from build123d import *

# Parameters (mm, degrees)
F0_R     = 6.35
F1_DEPTH = 4.7498
F2_R     = 3.175
F3_DEPTH = 25.4
F5_DEPTH = 0.381
F7_DEPTH = 0.381


with BuildPart() as f1:
    # F0 (on Right) → F1 (new body)
    with BuildSketch(Plane.YZ):
        Circle(F0_R)
    extrude(amount=F1_DEPTH)

    # F2 (on face) → F3 (cut)
    with BuildSketch(Plane.YZ.offset(4.7498)):
        Circle(F2_R)
    extrude(amount=-F3_DEPTH, mode=Mode.SUBTRACT)

    # F4 (on face) → F5 (cut)
    with BuildSketch(Plane(origin=(0, 0, 0), x_dir=(0, -1, 0), z_dir=(-1, 0, 0))):
        with BuildLine():
            ThreePointArc((0, -5.969), (4.22072, -4.22072), (5.969, 0))
            ThreePointArc((5.969, 0), (4.22072, 4.22072), (0, 5.969))
            ThreePointArc((0, 5.969), (-5.969, 0), (0, -5.969))
        make_face()
        with BuildLine():
            ThreePointArc((0, 3.556), (2.514472, 2.514472), (3.556, 0))
            ThreePointArc((3.556, 0), (2.514472, -2.514472), (0, -3.556))
            ThreePointArc((0, -3.556), (-3.556, 0), (0, 3.556))
        make_face(mode=Mode.SUBTRACT)
    extrude(amount=-F5_DEPTH, mode=Mode.SUBTRACT)

    # F6 (on face) → F7 (cut)
    with BuildSketch(Plane.YZ.offset(4.7498)):
        with BuildLine():
            ThreePointArc((0, -5.969), (4.22072, -4.22072), (5.969, 0))
            ThreePointArc((5.969, 0), (4.22072, 4.22072), (0, 5.969))
            ThreePointArc((0, 5.969), (-5.969, 0), (0, -5.969))
        make_face()
        with BuildLine():
            ThreePointArc((0, 3.556), (2.514472, 2.514472), (3.556, 0))
            ThreePointArc((3.556, 0), (2.514472, -2.514472), (0, -3.556))
            ThreePointArc((0, -3.556), (-3.556, 0), (0, 3.556))
        make_face(mode=Mode.SUBTRACT)
    extrude(amount=-F7_DEPTH, mode=Mode.SUBTRACT)


solid = f1.part
Source: CAD feature listing. Evaluate the final solid. Frame: model axes, mm. Round coordinates to 2 decimals unless told otherwise and drop trailing zeros. Write each loop counter-clockwise with the first axis right and the second up, starting at its lowest first coordinate (ties: lowest second). Pieces come first, ordered by that corner, then holes. Notation, with made-up numbers: M -39.75,80 L -5.75,80 A23 cw -5.75,108 Z; hole C -13.75,-19.75 d2. An arc over 180 degrees is marked long. One line per item, written item: value. Start each with the question number.
Item 1: Pin query (flat end, axial travel): pin 1 (6 mm diameter, centred on y = -1.5, z = -1, fed in from -X); pin 2 (1.5 mm diameter, centred on y = 5, z = -1, fed in from +X); pin 3 (1 mm diameter, centred on x = 2, y = -1, fed in from +Z). Return the tip coordinate at first contact, or that it passes through.
Item 2: Section query D-D (y = 4.25). Return the cut outline in (x, z), plus the area to 3 significant figures.
Item 3: Section query A-A (y = -2.5). Return the cut outline in (x, z), plus the area to 3 significant figures.
Item 4: Section query C-C (x = 0.85). Return the cut outline in (y, z) (3 decimals).
Item 5: Section query B-B (z = -0.5). Return the cut outline in (x, y), plus the area to 3 significant figures.
Item 6: Ray query, L1, parallel to Z at x = 2.9, y = 0 (3 decimals); L2, parallel to Y at x = 0.25, z = 0.25; L3, parallel to Z at x = 0.3, y = -2. Return the intervals inside material, ascending. Write a range as from..to.
Item 7: Mould query, pull axis Z, two halves, no side actions, for faces 1 (the cylindrical face through (2.34, -1.38, -6.2)), 2 (the flat face through (0.381, -3, -3)), 3 (the flat face through (4.369, 3, -3)). Classes: pulls with the +Z half, pulls with the -Z half, needs draft (parallel to the pull), parting line crosses it, or undercut.
Result set:
1. pin 1: stops at x = 0
1. pin 2: stops at x = 4.37
1. pin 3: stops at z = 6.33
2. outline: M 0,-4.72 L 4.75,-4.72 L 4.75,-4.19 L 4.37,-4.19 L 4.37,4.19 L 4.75,4.19 L 4.75,4.72 L 0,4.72 L 0,4.19 L 0.38,4.19 L 0.38,-4.19 L 0,-4.19 Z
2. area: 38.4 mm²
3. outline: M 0,-5.84 L 4.75,-5.84 L 4.75,-5.42 L 4.37,-5.42 L 4.37,-2.53 L 4.75,-2.53 L 4.75,-1.96 L 0,-1.96 L 0,-2.53 L 0.38,-2.53 L 0.38,-5.42 L 0,-5.42 Z; M 0,1.96 L 4.75,1.96 L 4.75,2.53 L 4.37,2.53 L 4.37,5.42 L 4.75,5.42 L 4.75,5.84 L 0,5.84 L 0,5.42 L 0.38,5.42 L 0.38,2.53 L 0,2.53 Z
3. area: 32.5 mm²
4. outline: C 0,0 d12.7; hole C 0,0 d6.35
5. outline: M 0,-6.33 L 4.75,-6.33 L 4.75,-5.95 L 4.37,-5.95 L 4.37,-3.52 L 4.75,-3.52 L 4.75,-3.14 L 0,-3.14 L 0,-3.52 L 0.38,-3.52 L 0.38,-5.95 L 0,-5.95 Z; M 0,3.14 L 4.75,3.14 L 4.75,3.52 L 4.37,3.52 L 4.37,5.95 L 4.75,5.95 L 4.75,6.33 L 0,6.33 L 0,5.95 L 0.38,5.95 L 0.38,3.52 L 0,3.52 Z
5. area: 26.7 mm²
6. L1: z = -6.35..-3.175, 3.175..6.35
6. L2: y = -6.35..-5.96, -3.55..-3.17, 3.17..3.55, 5.96..6.35
6. L3: z = -6.03..-5.62, -2.94..-2.47, 2.47..2.94, 5.62..6.03
7. face 1: parting line crosses it
7. face 2: undercut
7. face 3: undercut
